Design review of the part built by this model. Coordinates are the model's own, in mm. Coordinates: 2 decimals unless noted, no trailing zeros. Loops run counter-clockwise (first coordinate to the right, second up) from the corner with the lowest first, then second, coordinate; pieces in that order, holes last. Notation, with made-up numbers: M 14.5,38.25 L 47.5,38.25 A8 cw 47.5,43.25 Z; hole C 52,-25 d3. An arc over 180 degrees is marked long. Answer as a JSON object with one key per item and string values. Group by question number.
1. Consider section A-A (y = -18). State the section outline as (x, z) points, then the cut area to 3 significant figures.
2. Consider section C-C (x = -4). State the section outline as (y, z) points.
3. Consider section B-B (z = -0.35). State the section outline as (x, y) points.
4. To check wall thickness, follow probe 1 along X at (y, z) = (-21.5, -0.7); probe 2 along Y at (x, z) = (-13, -0.3); probe 3 along X at (y, z) = (21.5, 0.75). State the ranges of each line that lie inside material, in increasing order.
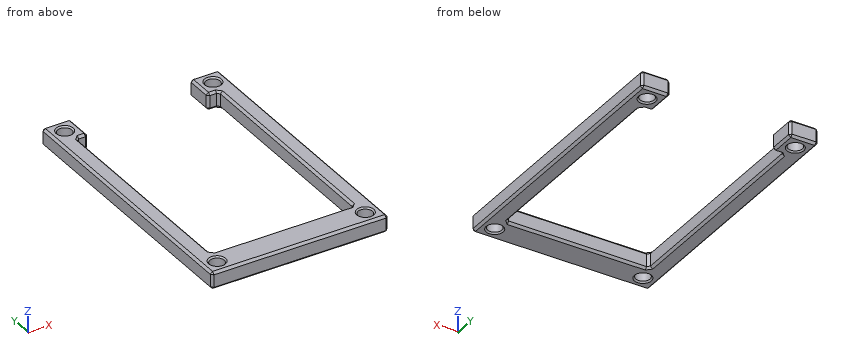
from build123d import *

# Parameters (mm, degrees)
AUFSATZ_LINEAR_AUSTRAGEN1_DEPTH           = 1.5
F_2_5_2_5_DURCHMESSER_BOHRUNG1_AT_2_COUNT = 2
F_2_5_2_5_DURCHMESSER_BOHRUNG1_AT_2_PITCH = 25.124689053
F_2_5_2_5_DURCHMESSER_BOHRUNG1_AT_3_COUNT = 2
F_2_5_2_5_DURCHMESSER_BOHRUNG1_AT_3_PITCH = 25.124689053
F_2_5_2_5_DURCHMESSER_BOHRUNG1_AT_4_COUNT = 2
F_2_5_2_5_DURCHMESSER_BOHRUNG1_AT_4_PITCH = 25.124689053
F_2_5_2_5_DURCHMESSER_BOHRUNG1_AT_5_COUNT = 2
F_2_5_2_5_DURCHMESSER_BOHRUNG1_AT_5_PITCH = 25.124689053
SKIZZE4_W                                 = 25
SKIZZE4_H                                 = 38
SCHNITT_LINEAR_AUSTRAGEN1_DEPTH           = 3
FASE1_SIZE                                = 0.4


with BuildPart() as part:
    # Skizze1 → Aufsatz-Linear austragen1 (new, symmetric)
    with BuildSketch(Plane(origin=(0, 0, 0), x_dir=(0, 1, 0), z_dir=(0, 0, 1))):
        Polygon((-24, 15.5), (24, 15.5), (24, 10.5), (-19, 10.5), (-19, -10.5), (24, -10.5), (24, -15.5), (-24, -15.5), align=None)
    extrude(amount=AUFSATZ_LINEAR_AUSTRAGEN1_DEPTH, both=True)

    # Skizze3 → Ø2.5 (2.5) Durchmesser Bohrung1 (revolve, cut)
    with BuildSketch(Plane(origin=(0, 0, 1.5), x_dir=(0, -1, 0), z_dir=(1, 0, 0))):
        Polygon((0, 0), (0, 3), (1.5, 3), (1.25, 2.75), (1.25, 0.25), (1.5, 0), align=None)
    f_2_5_2_5_durchmesser_bohrung1 = revolve(axis=Axis((0, 0, 7.85), (0, 0, -1)), mode=Mode.SUBTRACT)

    # Ø2.5 (2.5) Durchmesser Bohrung1 at 2: Ø2.5 (2.5) Durchmesser Bohrung1 ×2
    with Locations(*[Vector(0.5174193389091943, 0.8557319835805908, 0) * (i * F_2_5_2_5_DURCHMESSER_BOHRUNG1_AT_2_PITCH) for i in range(1, F_2_5_2_5_DURCHMESSER_BOHRUNG1_AT_2_COUNT)]):
        add(f_2_5_2_5_durchmesser_bohrung1, mode=Mode.SUBTRACT)

    # Ø2.5 (2.5) Durchmesser Bohrung1 at 3: Ø2.5 (2.5) Durchmesser Bohrung1 ×2
    with Locations(*[Vector(-0.5174193389091943, -0.8557319835805908, 0) * (i * F_2_5_2_5_DURCHMESSER_BOHRUNG1_AT_3_PITCH) for i in range(1, F_2_5_2_5_DURCHMESSER_BOHRUNG1_AT_3_COUNT)]):
        add(f_2_5_2_5_durchmesser_bohrung1, mode=Mode.SUBTRACT)

    # Ø2.5 (2.5) Durchmesser Bohrung1 at 4: Ø2.5 (2.5) Durchmesser Bohrung1 ×2
    with Locations(*[Vector(0.5174193389091946, -0.8557319835805907, 0) * (i * F_2_5_2_5_DURCHMESSER_BOHRUNG1_AT_4_PITCH) for i in range(1, F_2_5_2_5_DURCHMESSER_BOHRUNG1_AT_4_COUNT)]):
        add(f_2_5_2_5_durchmesser_bohrung1, mode=Mode.SUBTRACT)

    # Ø2.5 (2.5) Durchmesser Bohrung1 at 5: Ø2.5 (2.5) Durchmesser Bohrung1 ×2
    with Locations(*[Vector(-0.5174193389091944, 0.8557319835805907, 0) * (i * F_2_5_2_5_DURCHMESSER_BOHRUNG1_AT_5_PITCH) for i in range(1, F_2_5_2_5_DURCHMESSER_BOHRUNG1_AT_5_COUNT)]):
        add(f_2_5_2_5_durchmesser_bohrung1, mode=Mode.SUBTRACT)

    # Skizze4 → Schnitt-Linear austragen1 (cut)
    with BuildSketch(Plane.XY.offset(1.5)):
        Rectangle(SKIZZE4_W, SKIZZE4_H)
    extrude(amount=-SCHNITT_LINEAR_AUSTRAGEN1_DEPTH, mode=Mode.SUBTRACT)

    # Fase1
    fase1_edges = [part.edges().sort_by_distance(p)[0] for p in [
        (10.5, 21.5, -1.5),
        (13, 24, -1.5),
        (15.5, 0, -1.5),
        (0, -24, -1.5),
        (13, 24, 1.5),
        (-15.5, -24, 0),
        (-15.5, 24, 0),
        (-10.5, 24, 0),
        (10.5, 24, 0),
        (15.5, 24, 0),
        (15.5, -24, 0),
        (10.5, 21.5, 1.5),
        (0, -19, 1.5),
        (-13, 24, 1.5),
        (-15.5, 0, 1.5),
        (0, -24, 1.5),
        (-10.5, 21.5, -1.5),
        (-11.5, 19, -1.5),
        (-10.5, 21.5, 1.5),
        (11.5, 19, 1.5),
        (12.5, 0, 1.5),
        (-11.5, 19, 1.5),
        (-12.5, 0, 1.5),
        (12.5, -19, 0),
        (11.5, 19, -1.5),
        (10.5, 19, 0),
        (-10.5, 19, 0),
        (-12.5, 19, 0),
        (12.5, 0, -1.5),
        (12.5, 19, 0),
        (-12.5, 0, -1.5),
        (-12.5, -19, 0),
        (-15.5, 0, -1.5),
        (15.5, 0, 1.5),
        (-13, 24, -1.5),
        (0, -19, -1.5),
    ]]
    chamfer(fase1_edges, length=FASE1_SIZE)


solid = part.part
Findings below:
{
 "1": {"outline": "M -15.5,-1.1 L -15.1,-1.5 L -12.9,-1.5 L -12.5,-1.1 L -12.5,1.1 L -12.9,1.5 L -15.1,1.5 L -15.5,1.1 Z; M 12.5,-1.1 L 12.9,-1.5 L 15.1,-1.5 L 15.5,-1.1 L 15.5,1.1 L 15.1,1.5 L 12.9,1.5 L 12.5,1.1 Z", "area": "17.4 mm^2"},
 "2": {"outline": "M -24,-1.1 L -23.6,-1.5 L -19.4,-1.5 L -19,-1.1 L -19,1.1 L -19.4,1.5 L -23.6,1.5 L -24,1.1 Z"},
 "3": {"outline": "M -15.5,-23.6 L -15.1,-24 L 15.1,-24 L 15.5,-23.6 L 15.5,23.6 L 15.1,24 L 10.9,24 L 10.5,23.6 L 10.5,19.4 L 10.9,19 L 12.1,19 L 12.5,18.6 L 12.5,-18.6 L 12.1,-19 L -12.1,-19 L -12.5,-18.6 L -12.5,18.6 L -12.1,19 L -10.9,19 L -10.5,19.4 L -10.5,23.6 L -10.9,24 L -15.1,24 L -15.5,23.6 Z; hole C -13,-21.5 d2.5; hole C -13,21.5 d2.5; hole C 13,-21.5 d2.5; hole C 13,21.5 d2.5"},
 "4": {"probe 1": "x = -15.5 to -14.25, -11.75 to 11.75, 14.25 to 15.5", "probe 2": "y = -24 to -22.75, -20.25 to 20.25, 22.75 to 24", "probe 3": "x = -15.5 to -14.25, -11.75 to -10.5, 10.5 to 11.75, 14.25 to 15.5"}
}
